The listing builds one solid part. Answer for the finished solid, in the listing's coordinates (mm). A direction names the side the tool comes from. Round coordinates to 2 decimals unless told otherwise and drop trailing zeros. Write each loop counter-clockwise with the first axis right and the second up, starting at its lowest first coordinate (ties: lowest second). Pieces come first, ordered by that corner, then holes. Notation, with made-up numbers: (53.5, 7) - (63.5, 7) arc R25 cw to (63.5, 24) - close; hole circle Ø3 at (-34, 82.5). An arc over 180 degrees is marked (long way). Answer as CSV lines item,"result". Start each with the question number.
Item 1: A cutting plane is placed at B-B on z = 0. Determine the outline of the cut face in (x, y).
Item 2: A cutting plane is placed at A-A on x = 0. Determine the outline of the cut face in (y, z), and give its area (3 significant figures).
Item 3: Which of the six approach directions +Z, -Z, +X, -X, +Y, -Y give full straight-line access (tool end or side, diameter ignored) to faces 1 (the flat face through (1.1, 4.85, -1.1)), 2 (the flat face through (1, 6.7, 0)), 3 (the flat face through (0.3, 6, 0))?
Item 4: A cutting plane is placed at C-C on y = 2.25. Determine the outline of the cut face in (x, z), and give its area (3 significant figures).
Item 5: Straight lines are drawn through the part: line 1 along Y through (x, z) = (-0.2, 1.75); line 2 along Y through (x, z) = (-0.25, -0.35); line 3 along X through (y, z) = (6, 0.1). For each, find the intervals that lie inside material, in ascending order. Write a range as [from, to].
Item 6: Flat-ended cylindrical pins translate along their axes: pin 1 (1 mm diameter, centred on x = 0, y = 4.5, fed in from +Z); pin 2 (1 mm diameter, centred on y = 6.5, z = 1, fed in from +X); pin 3 (2 mm diameter, centred on x = -2, z = -1.5, fed in from -Y); pin 4 (3 mm diameter, centred on x = 2, y = 3, fed in from +Z). Find the tip coordinate at first contact, or state that the pin passes through.
```python
from build123d import *

# Parameters (mm, degrees)
SKETCH1_R               = 2.5
BOSS_EXTRUDE1_DEPTH     = 6.7
SKETCH2_OUTSIDE_W       = 8.948
SKETCH2_OUTSIDE_H       = 8.948
SKETCH2_OUTSIDE_R       = 0.85
CUT_EXTRUDE1_DEPTH      = 2
SKETCH3_OUTSIDE_W       = 8.948
SKETCH3_OUTSIDE_H       = 8.948
SKETCH3_OUTSIDE_R       = 1.25
CUT_EXTRUDE2_DEPTH      = 2.85
CHAMFER1_SIZE           = 0.2
SKETCH4_W               = 0.6
SKETCH4_H               = 0.9
CUT_EXTRUDE3_DEPTH      = 3.5
CUT_EXTRUDE3_DEPTH_BACK = 3.5
CHAMFER2_SIZE           = 0.25
FILLET1_R               = 0.1


with BuildPart() as part:
    # Sketch1 → Boss-Extrude1 (new body)
    with BuildSketch(Plane(origin=(0, 0, 0), x_dir=(1, 0, 0), z_dir=(0, 1, 0))):
        Circle(SKETCH1_R)
    extrude(amount=BOSS_EXTRUDE1_DEPTH)

    # Sketch2 outside → Cut-Extrude1 (cut)
    with BuildSketch(Plane.XZ):
        Rectangle(SKETCH2_OUTSIDE_W, SKETCH2_OUTSIDE_H)
        Circle(SKETCH2_OUTSIDE_R, mode=Mode.SUBTRACT)
    extrude(amount=-CUT_EXTRUDE1_DEPTH, mode=Mode.SUBTRACT)

    # Sketch3 outside → Cut-Extrude2 (cut)
    with BuildSketch(Plane.XZ.offset(-2)):
        Rectangle(SKETCH3_OUTSIDE_W, SKETCH3_OUTSIDE_H)
        Circle(SKETCH3_OUTSIDE_R, mode=Mode.SUBTRACT)
    extrude(amount=-CUT_EXTRUDE2_DEPTH, mode=Mode.SUBTRACT)

    # Chamfer1
    chamfer1_edges = [part.edges().sort_by_distance(p)[0] for p in [
        (-2.5, 6.7, 0),
    ]]
    chamfer(chamfer1_edges, length=CHAMFER1_SIZE)

    # Sketch4 → Cut-Extrude3 (cut, two sides)
    with BuildSketch(Plane.XY) as cut_extrude3_sk:
        with Locations((0, 6.25)):
            Rectangle(SKETCH4_W, SKETCH4_H)
    extrude(amount=CUT_EXTRUDE3_DEPTH, mode=Mode.SUBTRACT)
    extrude(cut_extrude3_sk.sketch, amount=-CUT_EXTRUDE3_DEPTH_BACK, mode=Mode.SUBTRACT)

    # Chamfer2
    chamfer2_edges = [part.edges().sort_by_distance(p)[0] for p in [
        (-0.85, 0, 0),
    ]]
    chamfer(chamfer2_edges, length=CHAMFER2_SIZE)

    # Fillet1
    fillet1_edges = [part.edges().sort_by_distance(p)[0] for p in [
        (-1.25, 4.85, 0),
    ]]
    fillet(fillet1_edges, radius=FILLET1_R)


solid = part.part
```
Geometry says:
1,outline,"(-2.5, 4.85) - (-1.35, 4.85) arc R0.1 cw to (-1.25, 4.75) - (-1.25, 2) - (-0.85, 2) - (-0.85, 0.25) - (-0.6, 0) - (0.6, 0) - (0.85, 0.25) - (0.85, 2) - (1.25, 2) - (1.25, 4.75) arc R0.1 cw to (1.35, 4.85) - (2.5, 4.85) - (2.5, 6.5) - (2.3, 6.7) - (0.3, 6.7) - (0.3, 5.8) - (-0.3, 5.8) - (-0.3, 6.7) - (-2.3, 6.7) - (-2.5, 6.5) - close"
2,outline,"(0, -0.6) - (0.25, -0.85) - (2, -0.85) - (2, -1.25) - (4.75, -1.25) arc R0.1 cw to (4.85, -1.35) - (4.85, -2.5) - (5.8, -2.5) - (5.8, 2.5) - (4.85, 2.5) - (4.85, 1.35) arc R0.1 cw to (4.75, 1.25) - (2, 1.25) - (2, 0.85) - (0.25, 0.85) - (0, 0.6) - close"
2,area,"15.2 mm^2"
3,face 1,"-Y"
3,face 2,"+Z, -Z, +X, -X, +Y"
3,face 3,"+Z, -Z, +Y"
4,outline,"circle Ø2.5 at (0, 0)"
4,area,"4.91 mm^2"
5,line 1,"y = [4.85, 5.8]"
5,line 2,"y = [0, 5.8]"
5,line 3,"x = [-2.5, -0.3], [0.3, 2.5]"
6,pin 1,"stops at z = 2.5"
6,pin 2,"stops at x = 2.45"
6,pin 3,"stops at y = 4.85"
6,pin 4,"stops at z = 1.15"
